Autodesk Inventor part; units mm, degrees
ref_plane "YZ Plane" through (0, 0, 0) normal (1, 0, 0) x (0, 1, 0)
ref_plane "XZ Plane" through (0, 0, 0) normal (0, 1, 0) x (-1, 0, 0)
ref_plane "XY Plane" through (0, 0, 0) normal (0, 0, 1) x (1, 0, 0)
sketch "Sketch1" plane through (0, 0, 0) normal (0, 0, 1) x (1, 0, 0)
  line L0 (31.5, 48.5) -> (31.5, -43.5)
  line L1 (31.5, -43.5) -> (-31.5, -43.5)
  line L2 (-31.5, -43.5) -> (-31.5, 48.5)
  line L3 (-31.5, 48.5) -> (31.5, 48.5)
  line L4 (25, -37) -> (25, 42) construction
  line L5 (25, 42) -> (-25, 42) construction
  line L6 (-25, 42) -> (-25, -37) construction
  line L7 (-25, -37) -> (25, -37) construction
  circle A0 centre (25, 42) radius 1.5
  circle A1 centre (25, -37) radius 1.5
  circle A2 centre (-25, -37) radius 1.5
  circle A3 centre (-25, 42) radius 1.5
  point P0 (0, 0)
  dimension "d0" = 5
extrude "Extrusion1" add sketch "Sketch1" along normal blind 3
properties part number "base teclado"
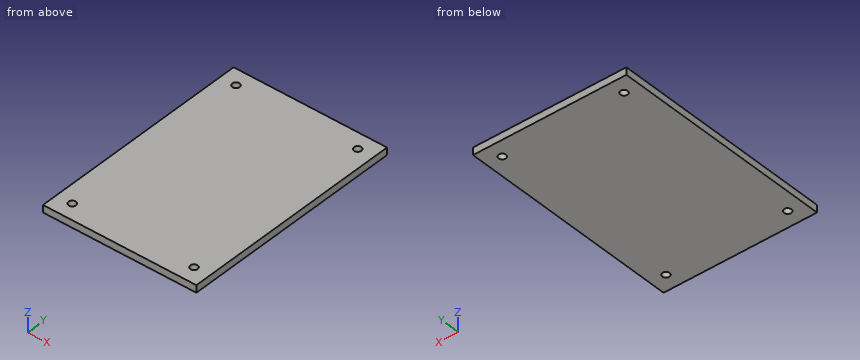
Could you check a few things on this model? Use its own coordinates, in mm. Round coordinates to 2 decimals unless told otherwise and drop trailing zeros. Write each loop counter-clockwise with the first axis right and the second up, starting at its lowest first coordinate (ties: lowest second). Pieces come first, ordered by that corner, then holes. Notation, with made-up numbers: M 58.25,34 L 80.25,34 A35 ccw 80.25,68 Z; hole C 10,-3.75 d1. An arc over 180 degrees is marked long. Answer in a Markdown table with one row per item. Add a question column.
Q1. Imagine slicing it at A-A (x = 25). Please give me the cut outline in (y, z), then the cut area to 3 significant figures.
Q2. Imagine slicing it at B-B (y = -37). Please give me the cut outline in (x, z), then the cut area to 3 significant figures.
Q3. Will this pin go through, and if not, where does the flat tip stop? pin 1 Ø2.5 at (x, y) = (-25, -37) entering from -Z.
Q4. If I drill on line 1 (Y direction, x = 25, z = 0.9), over which ranges is the centre line in solid material (lowest first)? Write a range as from..to.
Values:
| question | item | result |
|---|---|---|
| 1 | outline | M -43.5,0 L -38.5,0 L -38.5,3 L -43.5,3 Z; M -35.5,0 L 40.5,0 L 40.5,3 L -35.5,3 Z; M 43.5,0 L 48.5,0 L 48.5,3 L 43.5,3 Z |
| 1 | area | 258 mm^2 |
| 2 | outline | M -31.5,0 L -26.5,0 L -26.5,3 L -31.5,3 Z; M -23.5,0 L 23.5,0 L 23.5,3 L -23.5,3 Z; M 26.5,0 L 31.5,0 L 31.5,3 L 26.5,3 Z |
| 2 | area | 171 mm^2 |
| 3 | pin 1 | through |
| 4 | line 1 | -43.5..-38.5, -35.5..40.5, 43.5..48.5 |
